Verification items for the finished model (mm, model axes). A direction names the side the tool comes from. Coordinates: 2 decimals unless noted, no trailing zeros. Order: outer loops, then holes, each group sorted by start corner. A loop starts at its lowest first (then second) coordinate and runs counter-clockwise, first axis right, second up.
Q1. Thickness scan on line 1 (X direction, y = -13.25, z = -31.5); line 2 (Z direction, x = -3.5, y = -11.5) (3 decimals); line 3 (Z direction, x = -15, y = 2) (3 decimals). Record the ranges inside material, lowest first.
Q2. Cross-section at B-B, the plane z = 11. Record the boundary of the cut face in (x, y), and give its area (3 significant figures).
Q3. Depth check by flat-ended pin: P1, Ø1, axis at x = -20.5, y = -4, coming from the +Z side (3 decimals); P2, Ø2.5, axis at x = 5.5, y = -2.5, coming from the -Z side (3 decimals); P3, Ø9.5, axis at x = -18.5, z = 16, coming from the -Y side. Enter the tip coordinate at first touch or a pass-through.
Q4. Cross-section at A-A, the plane x = -11.5. Count the separate pieces of the cut face and the enclosed holes in it, and give its area (3 significant figures).
Q5. Draft check along Z on faces 4 (the cylindrical face through (1.7, -10.2, -67.28)), 5 (the flat face through (0, -6, -19.995)), 6 (the cylindrical face through (1.7, -10.2, 37.29)). Enter one of: pulls with the +Z half, pulls with the -Z half, needs draft (parallel to the pull), parting line crosses it, or undercut.
Q6. Set-up check for faces 1 (the flat face through (1.537, -8.619, -15.065)), 2 (the cylindrical face through (-16.3, -10.2, -67.28)), 3 (the flat face through (-21, -3, -56.995)): record each of +Z, -Z, +X, -X, +Y, -Y from which the full face is reachable in a straight line by a thin tool's end or side.
from build123d import *
from OCP.BRepFilletAPI import BRepFilletAPI_MakeChamfer

# Parameters (mm, degrees)
SKETCH1_W           = 30
SKETCH1_H           = 130
SKETCH1_R           = 2.5
BOSS_EXTRUDE1_DEPTH = 3
SKETCH2_W           = 30
SKETCH2_H           = 12
BOSS_EXTRUDE2_DEPTH = 12
CUT_EXTRUDE1_REACH  = 88.274
SKETCH3_R           = 4
FILLET1_R           = 6
SKETCH4_R           = 4
CUT_EXTRUDE2_DEPTH  = 19
SKETCH5_W           = 6
SKETCH5_H           = 84
SKETCH5_H_2         = 11
BOSS_EXTRUDE3_DEPTH = 6
CHAMFER1_SIZE       = 6
BOSS_EXTRUDE4_DEPTH = 6
SKETCH7_W           = 12
SKETCH7_H           = 10
BOSS_EXTRUDE5_DEPTH = 17
CHAMFER2_SIZE       = 17
CHAMFER2_SIZE2      = 12


with BuildPart() as part:
    # Sketch1 → Boss-Extrude1 (new body)
    with BuildSketch(Plane(origin=(0, 0, 0), x_dir=(1, 0, 0), z_dir=(0, 1, 0))):
        with Locations((-7.37923135, 14.994995261)):
            Rectangle(SKETCH1_W, SKETCH1_H)
        with Locations(Location((-16.37923135, -24.005004739, 0), (0, 0, 270))):
            Circle(SKETCH1_R, mode=Mode.SUBTRACT)
        with Locations(Location((1.62076865, -24.005004739, 0), (0, 0, 270))):
            Circle(SKETCH1_R, mode=Mode.SUBTRACT)
        with Locations(Location((1.62076865, -42.005004739, 0), (0, 0, 270))):
            Circle(SKETCH1_R, mode=Mode.SUBTRACT)
        with Locations(Location((-16.37923135, -42.005004739, 0), (0, 0, 270))):
            Circle(SKETCH1_R, mode=Mode.SUBTRACT)
        with Locations(Location((-16.37923135, 71.994995261, 0), (0, 0, 270))):
            Circle(SKETCH1_R, mode=Mode.SUBTRACT)
        with Locations(Location((-16.37923135, 53.994995261, 0), (0, 0, 270))):
            Circle(SKETCH1_R, mode=Mode.SUBTRACT)
        with Locations(Location((1.62076865, 71.994995261, 0), (0, 0, 270))):
            Circle(SKETCH1_R, mode=Mode.SUBTRACT)
        with Locations(Location((1.62076865, 53.994995261, 0), (0, 0, 270))):
            Circle(SKETCH1_R, mode=Mode.SUBTRACT)
    extrude(amount=BOSS_EXTRUDE1_DEPTH)

    # Sketch2 → Boss-Extrude2 (add)
    with BuildSketch(Plane.XZ):
        with Locations((-7.37923135, -62.994995261)):
            Rectangle(SKETCH2_W, SKETCH2_H)
        with Locations((-7.37923135, 33.005004739)):
            Rectangle(SKETCH2_W, SKETCH2_H)
    extrude(amount=BOSS_EXTRUDE2_DEPTH)

    # Sketch3 → Cut-Extrude1 (cut, up to next)
    with BuildSketch(Plane(origin=(7.62076865, 0, 0), x_dir=(0, 0, -1), z_dir=(1, 0, 0)), mode=Mode.PRIVATE) as cut_extrude1_sk1:
        with Locations((-33.005004739, -6)):
            Circle(SKETCH3_R)
    cut_extrude1_tool1 = extrude(cut_extrude1_sk1.sketch, amount=-CUT_EXTRUDE1_REACH, mode=Mode.PRIVATE) & part.part
    # Sketch3 → Cut-Extrude1 (cut, up to next)
    with BuildSketch(Plane(origin=(7.62076865, 0, 0), x_dir=(0, 0, -1), z_dir=(1, 0, 0)), mode=Mode.PRIVATE) as cut_extrude1_sk2:
        with Locations((62.994995261, -6)):
            Circle(SKETCH3_R)
    cut_extrude1_tool2 = extrude(cut_extrude1_sk2.sketch, amount=-CUT_EXTRUDE1_REACH, mode=Mode.PRIVATE) & part.part
    add(cut_extrude1_tool1.solids().sort_by_distance((7.620769, -6, 33.005005))[0], mode=Mode.SUBTRACT)
    add(cut_extrude1_tool2.solids().sort_by_distance((7.620769, -6, -62.994995))[0], mode=Mode.SUBTRACT)

    # Fillet1
    fillet1_edges = [part.edges().sort_by_distance(p)[0] for p in [
        (-7.37923135, -12, -68.994995261),
        (-7.37923135, -12, -56.994995261),
        (-7.37923135, -12, 27.005004739),
        (-7.37923135, -12, 39.005004739),
    ]]
    fillet(fillet1_edges, radius=FILLET1_R - 0.0001)  # a hair under: the kernel refuses the full size

    # Sketch4 → Cut-Extrude2 (cut)
    with BuildSketch(Plane.XZ):
        with Locations((-16.37923135, -53.994995261)):
            Circle(SKETCH4_R)
        with Locations((-16.37923135, -71.994995261)):
            Circle(SKETCH4_R)
        with Locations((1.62076865, -71.994995261)):
            Circle(SKETCH4_R)
        with Locations((1.62076865, -3.994995261)):
            Circle(SKETCH4_R)
        with Locations((1.62076865, 24.005004739)):
            Circle(SKETCH4_R)
        with Locations((-16.37923135, 24.005004739)):
            Circle(SKETCH4_R)
        with Locations((-16.37923135, 42.005004739)):
            Circle(SKETCH4_R)
        with Locations((1.62076865, 42.005004739)):
            Circle(SKETCH4_R)
    extrude(amount=CUT_EXTRUDE2_DEPTH, mode=Mode.SUBTRACT)

    # Sketch5 → Boss-Extrude3 (add)
    with BuildSketch(Plane.XZ):
        with Locations((-7.37923135, -14.994995261)):
            Rectangle(SKETCH5_W, SKETCH5_H)
        with Locations((-7.37923135, -74.494995261)):
            Rectangle(SKETCH5_W, SKETCH5_H_2)
        with Locations((-7.37923135, 44.505004739)):
            Rectangle(SKETCH5_W, SKETCH5_H_2)
    extrude(amount=BOSS_EXTRUDE3_DEPTH)

    # Chamfer1
    chamfer1_edges = [part.edges().sort_by_distance(p)[0] for p in [
        (-7.37923135, -6, -79.994995261),
        (-7.37923135, -6, 50.005004739),
    ]]
    chamfer(chamfer1_edges, length=CHAMFER1_SIZE)

    # Sketch6 → Boss-Extrude4 (add)
    with BuildSketch(Plane.ZY.offset(10.37923135)):
        with BuildLine():
            Line((-62.994995261, -17), (33.005004739, -17))
            ThreePointArc((33.005004739, -17), (40.783179332, -13.778174593), (44.005004739, -6))
            Line((44.005004739, -6), (39.005004739, -6))
            ThreePointArc((39.005004739, -6), (33.005004739, -12), (27.005004739, -6))
            Line((27.005004739, -6), (-56.994995261, -6))
            ThreePointArc((-56.994995261, -6), (-62.994995261, -12), (-68.994995261, -6))
            Line((-68.994995261, -6), (-73.994995261, -6))
            ThreePointArc((-73.994995261, -6), (-70.773169854, -13.778174593), (-62.994995261, -17))
        make_face()
    extrude(amount=-BOSS_EXTRUDE4_DEPTH)

    # Sketch7 → Boss-Extrude5 (add)
    with BuildSketch(Plane.XZ):
        with Locations((-16.37923135, -14.994995261)):
            Rectangle(SKETCH7_W, SKETCH7_H)
        with Locations((1.62076865, -14.994995261)):
            Rectangle(SKETCH7_W, SKETCH7_H)
    extrude(amount=BOSS_EXTRUDE5_DEPTH)

    # Chamfer2: one chamfer whose edges measure the first distance from different faces: ONE call of the kernel's chamfer builder (chamfer() names one face for all edges)
    chamfer2_edges_1 = [part.edges().sort_by_distance(p)[0] for p in [
        (-22.37923135, -17, -14.994995261),
    ]]
    chamfer2_side_1 = [part.faces().sort_by_distance(p)[0] for p in [
        (-22.37923135, -2.310192331, -14.994995261),
    ]]
    chamfer2_edges_2 = [part.edges().sort_by_distance(p)[0] for p in [
        (7.62076865, -17, -14.994995261),
    ]]
    chamfer2_side_2 = [part.faces().sort_by_distance(p)[0] for p in [
        (7.62076865, -2.310192331, -14.994995261),
    ]]
    chamfer2 = BRepFilletAPI_MakeChamfer(part.part.solid().wrapped)
    for e in chamfer2_edges_1:
        chamfer2.Add(CHAMFER2_SIZE, CHAMFER2_SIZE2, e.wrapped, chamfer2_side_1[0].wrapped)  # the first distance lies on this face
    for e in chamfer2_edges_2:
        chamfer2.Add(CHAMFER2_SIZE, CHAMFER2_SIZE2, e.wrapped, chamfer2_side_2[0].wrapped)  # the first distance lies on this face
    add(Compound.cast(chamfer2.Shape()), mode=Mode.REPLACE)


solid = part.part
Check values:
1. line 1: x = -10.38 to -4.38
1. line 2: z = -65.393 to -60.597, -19.995 to -9.995, 30.607 to 35.403
1. line 3: z = -79.995 to -74.08, -69.91 to -56.08, -51.91 to 21.92, 26.09 to 39.92, 44.09 to 50.005
2. outline: (-22.38, 0) - (-10.38, 0) - (-10.38, -17) - (-4.38, -17) - (-4.38, 0) - (7.62, 0) - (7.62, 3) - (-22.38, 3) - close
2. area: 192 mm2
3. P1: stops at z = 39.005
3. P2: stops at z = -68.995
3. P3: stops at y = 0
4. separate pieces: 1
4. enclosed holes: 2
4. area: 701 mm2
5. face 4: pulls with the -Z half
5. face 5: undercut
5. face 6: pulls with the +Z half
6. face 1: +X, -Y
6. face 2: -Z, -X, -Y
6. face 3: -X, -Y
